For this review, take the finished solid that the model builds, in its own axes (mm). Face numbers are marked on the shaded views. A direction names the side the tool comes from. Round coordinates to 2 decimals unless told otherwise and drop trailing zeros. Order: outer loops, then holes, each group sorted by start corner. A loop starts at its lowest first (then second) coordinate and runs counter-clockwise, first axis right, second up. Notation, with made-up numbers: M -1.75,37 L 20.25,37 A25 cw 20.25,62 Z; hole C 31,2.5 d3. An arc over 180 degrees is marked long. Put each result on its own line as item: value.
Autodesk Inventor part; units mm, degrees
ref_plane "YZ Plane" through (0, 0, 0) normal (1, 0, 0) x (0, 1, 0)
ref_plane "XZ Plane" through (0, 0, 0) normal (0, 1, 0) x (-1, 0, 0)
ref_plane "XY Plane" through (0, 0, 0) normal (0, 0, 1) x (1, 0, 0)
sketch "Эскиз1" plane through (0, 0, 0) normal (0, 1, 0) x (-1, 0, 0)
  line L0 (-75, 75) -> (75, 75)
  line L1 (75, 75) -> (75, -75)
  line L2 (75, -75) -> (-75, -75)
  line L3 (-75, -75) -> (-75, 75)
  line L4 (-75, 75) -> (75, -75) construction
  line L5 (75, 75) -> (-75, -75) construction
  point P0 (0, 0)
  dimension "d0" = 150
  dimension "d1" = 150
extrude "Выдавливание1" add sketch "Эскиз1" along normal blind 10
sketch "Эскиз2" plane through (0, 10, 0) normal (0, 1, 0) x (1, 0, 0)
  circle A0 centre (0, 0) radius 75
  circle A1 centre (0, 0) radius 65
  dimension "d4" = 150
  dimension "d5" = 130
extrude "Выдавливание2" add sketch "Эскиз2" along normal blind 160
sketch "Эскиз3" plane through (0, 10, 0) normal (0, 1, 0) x (1, 0, 0)
  line L0 (0, 0) -> (-53.033, -53.033)
  arc A0 (-75, 0) -> (0, -75) centre (0, 0) ccw
  line L1 (0, 0) -> (75, 0) construction
  line L2 (-53.033, -53.033) -> (-66.033, -53.033)
  line L3 (-66.033, -53.033) -> (-66.033, -66.033)
  line L4 (-66.033, -66.033) -> (-53.033, -66.033)
  line L5 (-53.033, -66.033) -> (-53.033, -53.033)
  line L6 (-53.033, -66.033) -> (-35.5618, -66.033)
  line L7 (-66.033, -53.033) -> (-66.033, -35.5618)
  arc A1 (-66.033, -35.5618) -> (-35.5618, -66.033) centre (0, 0) ccw
  circle A2 centre (-59.533, -59.533) radius 3
  dimension "d8" = 135
  dimension "d9" = 13
  dimension "d10" = 13
  dimension "d11" = 6
  dimension "d12" = 6.5
  dimension "d13" = 6.5
extrude "Выдавливание3" add sketch "Эскиз3" along normal up to surface (160 mm away)
pattern_circular "Круговой массив1" count 4 over 360 about axis through (0, 10, 0) along (0, 1, 0) of "Выдавливание3"
sketch "Эскиз5" plane through (0, 170, 0) normal (0, 1, 0) x (1, 0, 0)
  line L0 (75, 0) -> (75, 75)
  line L1 (75, 35.8218) -> (45, 35.8218)
  line L2 (45, 35.8218) -> (45, -35.5618)
  line L3 (45, -35.5618) -> (75, -35.5618)
  line L4 (75, -35.5618) -> (75, 35.8218)
  point P0 (0, 0)
  dimension "d21" = 30
extrude "Выдавливание5" cut sketch "Эскиз5" against normal up to surface (160 mm away)
sketch "Эскиз6" plane through (0, 170, 0) normal (0, 1, 0) x (1, 0, 0)
  line L0 (66.033, 66.033) -> (66.033, 35.8218)
  line L1 (66.033, 35.8218) -> (36.033, 35.8218)
  line L2 (36.033, 35.8218) -> (36.033, 45.8218)
  line L3 (36.033, 45.8218) -> (66.033, 45.8218)
  line L4 (66.033, 45.8218) -> (66.033, 35.8218)
  arc A0 (54.2384, 35.8218) -> (54.4092, -35.5618) centre (0, 0) ccw
  line L5 (36.033, 45.8218) -> (46.6128, 45.8218)
  line L6 (66.033, -35.5618) -> (66.033, -66.033)
  line L7 (66.033, -35.5618) -> (36.033, -35.5618)
  line L8 (36.033, -35.5618) -> (36.033, -45.5618)
  line L9 (36.033, -45.5618) -> (66.033, -45.5618)
  line L10 (66.033, -45.5618) -> (66.033, -35.5618)
  line L11 (36.033, 45.8218) -> (41.033, 45.8218)
  line L12 (41.033, 45.8218) -> (41.033, -45.5618)
  line L13 (41.033, -45.5618) -> (36.033, -45.5618)
  line L14 (36.033, -45.5618) -> (36.033, 45.8218)
  dimension "d24" = 30
  dimension "d25" = 10
  dimension "d26" = 30
  dimension "d27" = 10
  dimension "d28" = 5
extrude "Выдавливание6" add sketch "Эскиз6" against normal up to surface (160 mm away) contours L0 L1 A0 L3 | L1 L12 L3 A0 | L12 L7 L14 L1 | L1 L2 L3 L12 | L9 L12 L7 A0 | A0 L7 L6 L9 | L12 L9 L8 L7
sketch "Эскиз7" plane through (41.033, 170, 35.5618) normal (1, 0, 0) x (0, 0, -1)
  point P0 (35.5618, -170)
sketch "Эскиз8" plane through (41.033, 170, 35.5618) normal (1, 0, 0) x (0, 0, -1)
  circle A0 centre (31.3816, -91.5) radius 2.1
  line L0 (33.0222, -106.4854) -> (32.894, -106.0661)
  arc A1 (33.0222, -106.4854) -> (33.2588, -106.8521) centre (33.7873, -106.2515) ccw
  line L1 (34.1201, -107.61) -> (33.2588, -106.8521)
  line L2 (34.3916, -117.7894) -> (34.3916, -108.2106)
  arc A2 (34.3916, -108.2106) -> (34.1201, -107.61) centre (33.5916, -108.2106) ccw
  arc A3 (34.1201, -118.39) -> (34.3916, -117.7894) centre (33.5916, -117.7894) ccw
  line L3 (33.2588, -119.1479) -> (34.1201, -118.39)
  line L4 (32.894, -119.9339) -> (33.0222, -119.5146)
  arc A4 (33.2588, -119.1479) -> (33.0222, -119.5146) centre (33.7873, -119.7485) ccw
  arc A5 (32.129, -120.5) -> (32.894, -119.9339) centre (32.129, -119.7) ccw
  line L5 (29.6416, -120.5) -> (32.129, -120.5)
  arc A6 (28.8416, -119.7) -> (29.6416, -120.5) centre (29.6416, -119.7) ccw
  line L6 (28.8416, -106.3) -> (28.8416, -119.7)
  arc A7 (29.6416, -105.5) -> (28.8416, -106.3) centre (29.6416, -106.3) ccw
  line L7 (32.129, -105.5) -> (29.6416, -105.5)
  arc A8 (32.894, -106.0661) -> (32.129, -105.5) centre (32.129, -106.3) ccw
  line L8 (34.2451, -137.4464) -> (33.688, -138.0036)
  line L9 (32.6416, -138.15) -> (33.3345, -138.15)
  arc A9 (33.3345, -138.15) -> (33.688, -138.0036) centre (33.3345, -137.65) ccw
  arc A10 (32.1416, -137.65) -> (32.6416, -138.15) centre (32.6416, -137.65) ccw
  line L10 (32.1416, -131.15) -> (32.1416, -137.65)
  arc A11 (32.6416, -130.65) -> (32.1416, -131.15) centre (32.6416, -131.15) ccw
  line L11 (33.3345, -130.65) -> (32.6416, -130.65)
  line L12 (33.688, -130.7964) -> (34.2451, -131.3536)
  arc A12 (33.688, -130.7964) -> (33.3345, -130.65) centre (33.3345, -131.15) ccw
  arc A13 (34.3916, -131.7071) -> (34.2451, -131.3536) centre (33.8916, -131.7071) ccw
  line L13 (34.3916, -142.5) -> (34.3916, -62.5)
  line L14 (28.8416, -113) -> (34.3916, -113)
  line L15 (24.1166, -123) -> (39.1166, -123)
  line L16 (39.1166, -123) -> (39.1166, -103)
  line L17 (39.1166, -103) -> (24.1166, -103)
  line L18 (24.1166, -103) -> (24.1166, -123)
  line L19 (24.1166, -123) -> (39.1166, -103) construction
  line L20 (39.1166, -123) -> (24.1166, -103) construction
  line L21 (30.3345, -139.4) -> (36.3345, -139.4)
  line L22 (36.3345, -139.4) -> (36.3345, -129.4)
  line L23 (36.3345, -129.4) -> (30.3345, -129.4)
  line L24 (30.3345, -129.4) -> (30.3345, -139.4)
  line L25 (30.3345, -139.4) -> (36.3345, -129.4) construction
  line L26 (36.3345, -139.4) -> (30.3345, -129.4) construction
  circle A14 centre (31.3816, -91.5) radius 5
  circle A15 centre (31.3816, -91.5) radius 2.1
  line L27 (33.0222, -106.4854) -> (32.894, -106.0661)
  arc A16 (33.0222, -106.4854) -> (33.2588, -106.8521) centre (33.7873, -106.2515) ccw
  line L28 (34.1201, -107.61) -> (33.2588, -106.8521)
  line L29 (34.3916, -117.7894) -> (34.3916, -108.2106)
  arc A17 (34.3916, -108.2106) -> (34.1201, -107.61) centre (33.5916, -108.2106) ccw
  arc A18 (34.1201, -118.39) -> (34.3916, -117.7894) centre (33.5916, -117.7894) ccw
  line L30 (33.2588, -119.1479) -> (34.1201, -118.39)
  line L31 (32.894, -119.9339) -> (33.0222, -119.5146)
  arc A19 (33.2588, -119.1479) -> (33.0222, -119.5146) centre (33.7873, -119.7485) ccw
  arc A20 (32.129, -120.5) -> (32.894, -119.9339) centre (32.129, -119.7) ccw
  line L32 (29.6416, -120.5) -> (32.129, -120.5)
  arc A21 (28.8416, -119.7) -> (29.6416, -120.5) centre (29.6416, -119.7) ccw
  line L33 (28.8416, -106.3) -> (28.8416, -119.7)
  arc A22 (29.6416, -105.5) -> (28.8416, -106.3) centre (29.6416, -106.3) ccw
  line L34 (32.129, -105.5) -> (29.6416, -105.5)
  arc A23 (32.894, -106.0661) -> (32.129, -105.5) centre (32.129, -106.3) ccw
  line L35 (34.2451, -137.4464) -> (33.688, -138.0036)
  line L36 (32.6416, -138.15) -> (33.3345, -138.15)
  arc A24 (33.3345, -138.15) -> (33.688, -138.0036) centre (33.3345, -137.65) ccw
  arc A25 (32.1416, -137.65) -> (32.6416, -138.15) centre (32.6416, -137.65) ccw
  line L37 (32.1416, -131.15) -> (32.1416, -137.65)
  arc A26 (32.6416, -130.65) -> (32.1416, -131.15) centre (32.6416, -131.15) ccw
  line L38 (33.3345, -130.65) -> (32.6416, -130.65)
  line L39 (33.688, -130.7964) -> (34.2451, -131.3536)
  arc A27 (33.688, -130.7964) -> (33.3345, -130.65) centre (33.3345, -131.15) ccw
  arc A28 (34.3916, -131.7071) -> (34.2451, -131.3536) centre (33.8916, -131.7071) ccw
  line L40 (34.3916, -142.5) -> (34.3916, -62.5)
  line L41 (28.8416, -113) -> (34.3916, -113)
  line L42 (24.1166, -123) -> (39.1166, -123)
  line L43 (39.1166, -123) -> (39.1166, -103)
  line L44 (39.1166, -103) -> (24.1166, -103)
  line L45 (24.1166, -103) -> (24.1166, -123)
  line L46 (24.1166, -123) -> (39.1166, -103) construction
  line L47 (39.1166, -123) -> (24.1166, -103) construction
  line L48 (30.3345, -139.4) -> (36.3345, -139.4)
  line L49 (36.3345, -139.4) -> (36.3345, -129.4)
  line L50 (36.3345, -129.4) -> (30.3345, -129.4)
  line L51 (30.3345, -129.4) -> (30.3345, -139.4)
  line L52 (30.3345, -139.4) -> (36.3345, -129.4) construction
  line L53 (36.3345, -139.4) -> (30.3345, -129.4) construction
  circle A29 centre (31.3816, -91.5) radius 5
  point P0 (35.5618, -170)
  point P1 (31.6166, -113)
  point P2 (33.3345, -134.4)
  point P3 (31.6166, -113)
  point P4 (33.3345, -134.4)
  dimension "d31" = 15
  dimension "d32" = 20
  dimension "d33" = 6
  dimension "d34" = 10
  dimension "d35" = 10
  dimension "d36" = 15
  dimension "d37" = 20
  dimension "d38" = 6
  dimension "d39" = 10
  dimension "d40" = 10
extrude "Выдавливание7" cut sketch "Эскиз8" against normal blind 10 contours A0 | A1 L1 A2 L2 L14 L6 A7 L7 A8 L0 | L0 A8 L7 A7 L6 A6 L5 A5 L4 A4 L3 A3 L13 L15 L18 L17 A2 L1 A1 | L13 L17 L16 L15 L2 | L2 A3 L3 A4 L4 A5 L5 A6 L6 L14 | A14 L13 | L13 A14 | L23 L22 L21 L13 | L13 L21 L24 L23
chamfer "Фаска1" distance 10 angle 45 2 edges at (46.3586, 90, 45.5618) (46.1017, 90, -45.8218)
properties part number "000.201 - Станина" material "Пластик АБС"
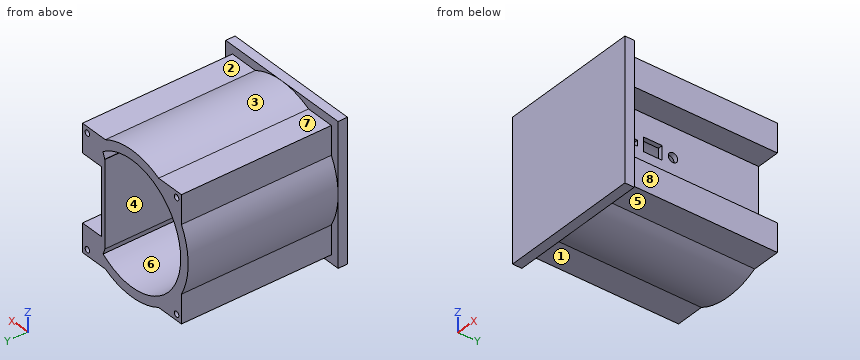
(1) Insertion check: pin 1 Ø9 at (y, z) = (99.5, -52) entering from +X; pin 2 Ø12 at (y, z) = (92, 12) entering from +X; pin 3 Ø2 at (y, z) = (94, 48) entering from -X. Each pin has a flat end and moves straight along its axis. Give the tip position at first contact, or say it passes through.
A:
pin 1: stops at x = 66.03
pin 2: stops at x = 41.03
pin 3: stops at x = -66.03
(2) To check wall thickness, follow L1, parallel to Z at x = 0, y = 50.5; L2, parallel to X at y = 133.5, z = -1; L3, parallel to Z at x = 40, y = 78. State the ranges of each line that lie inside material, in increasing order.
A:
L1: z = -75 to -65, 65 to 75
L2: x = -74.99 to -64.99, 36.03 to 41.03
L3: z = -66.03 to -0.79, 9.16 to 66.03
(3) Add section D-D on x = 3.5. Give the boundary of the cut face in (y, z).
A:
outline: M 0,-75 L 10,-75 L 10,-74.92 L 170,-74.92 L 170,-64.91 L 10,-64.91 L 10,64.91 L 170,64.91 L 170,74.92 L 10,74.92 L 10,75 L 0,75 Z
(4) Add section A-A on y = 78.5. Give the boundary of the cut face in (x, z).
A:
outline: M -66.03,-66.03 L -35.56,-66.03 A75 ccw 35.56,-66.03 L 66.03,-66.03 L 66.03,-35.82 L 41.03,-35.82 L 41.03,-0.82 L 36.03,-0.82 L 36.03,-45.82 L 36.1,-45.82 L 38.53,-52.35 A65 cw long 38.82,52.13 L 36.36,45.56 L 36.03,45.56 L 36.03,9.18 L 41.03,9.18 L 41.03,35.56 L 66.03,35.56 L 66.03,66.03 L 35.56,66.03 A75 ccw -35.56,66.03 L -66.03,66.03 L -66.03,35.56 A75 ccw -66.03,-35.56 Z; hole C -59.53,-59.53 d6; hole C -59.53,59.53 d6; hole C 59.53,-59.53 d6; hole C 59.53,59.53 d6
(5) Add section C-C on y = 12.5. Give the boundary of the cut face in (x, z), then the cut area to 3 significant figures.
A:
outline: M -66.03,-66.03 L -35.56,-66.03 A75 ccw 35.56,-66.03 L 66.03,-66.03 L 66.03,-35.82 L 41.03,-35.82 L 41.03,35.56 L 66.03,35.56 L 66.03,66.03 L 35.56,66.03 A75 ccw -35.56,66.03 L -66.03,66.03 L -66.03,35.56 A75 ccw -66.03,-35.56 Z; hole C -59.53,-59.53 d6; hole C -59.53,59.53 d6; hole M 36.03,-45.82 L 36.03,45.56 L 36.36,45.56 L 38.82,52.13 A65 ccw long 38.53,-52.35 L 36.1,-45.82 Z; hole C 59.53,-59.53 d6; hole C 59.53,59.53 d6
area: 5,740 mm2
(6) Draft analysis for pull direction Z (two halves, no side actions). For the marked faces 6, 7 and 8, state which applies: released by +Z, released by -Z, zero draft, split by the parting line, or undercut.
A:
face 6: undercut
face 7: released by +Z
face 8: zero draft
(7) For the marked faces 1, 2, 3, 4 and 5, list the 3-axis set-ups (+Z, -Z, +X, -X, +Y, -Y) from which the entire face can be reached by the end or side of a thin tool; tool diameter is ignored.
A:
face 1: -Z, -X, +Y
face 2: +Z, +X, +Y
face 3: +Z, +Y
face 4: +Y
face 5: -Z, +X, +Y
(8) Add section B-B on z = 27. Give the boundary of the cut face in (x, y), then the cut area to 3 significant figures.
A:
outline: M -75,0 L 75,0 L 75,10 L 41.03,10 L 41.03,170 L 36.03,170 L 36.03,10 L -59.13,10 L -59.13,170 L -69.97,170 L -69.97,10 L -75,10 Z
area: 4,040 mm2
